Input: part model. Units: mm. Frame: model coordinates. Face numbers are marked on the shaded views. A direction names the side the tool comes from. Coordinates: 2 decimals unless noted, no trailing zeros. Write each loop counter-clockwise with the first axis right and the second up, starting at its lowest first coordinate (ties: lowest second). Pieces come first, ordered by that corner, then holes. Notation, with made-up numbers: (17, 70.25) -> (21, 70.25) arc R11 cw to (21, 91.25) -> close; hole circle Ø8 at (87.5, 30). An arc over 180 degrees is marked (long way). Use one line per item in the form item = value. Start each with the question number.
(1) Ray query, line 1 along Z through (x, y) = (0.05, -24.13) (3 decimals); line 2 along X through (y, z) = (-22.5, 2); line 3 along Y through (x, z) = (2.25, 0.75). Return the intervals inside material, ascending.
(2) Set-up query: the marked faces 1, 2, 3, 4 and 5. Return all of +Z, -Z, +X, -X, +Y, -Y with unobstructed straight access to the full face (end or side cutting, diameter ignored); none if empty.
(3) Cut plane B-B on x = -1.25. Return the cut outline in (y, z) (3 decimals), plus the area to 3 significant figures.
(4) Cut plane C-C on z = -1. Return the cut outline in (x, y), plus the area to 3 significant figures.
(5) Cut plane D-D on y = -9.5. Return the cut outline in (x, z).
(6) First-contact query: pin 1 (1.5 mm diameter, centred on y = -24.13, z = 0, fed in from +X); pin 2 (1.6 mm diameter, centred on y = -21, z = 0, fed in from -X); pin 3 (1 mm diameter, centred on x = 0, z = 3.5, fed in from -Y). Flat tips, straight axial feed; report the tip coordinate or a pass-through.
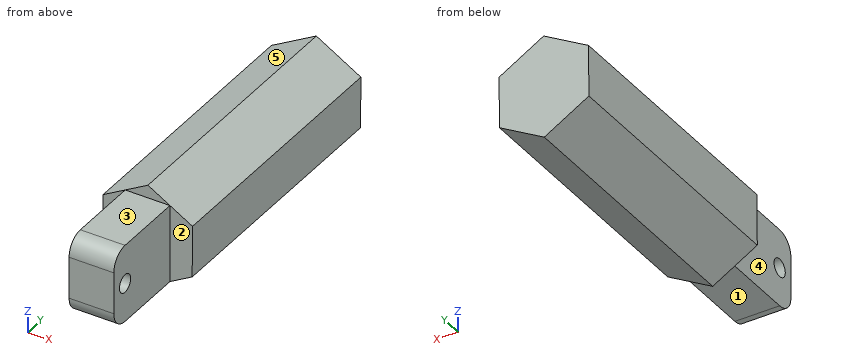
```python
from build123d import *

# Parameters (mm, degrees)
F1_DEPTH = 19.05
F2_W     = 3.175
F2_H     = 5.499398
F3_DEPTH = 6.35
F4_R     = 1.27
F6_D     = 1.27
F6_DEPTH = 25.4


with BuildPart() as f1:
    # F0 (on Front) → F1 (new body)
    with BuildSketch(Plane.XZ):
        Polygon((3.186096, 1.813733), (0.022309, 3.666106), (-3.163787, 1.852373), (-3.186096, -1.813733), (-0.022309, -3.666106), (3.163787, -1.852373), align=None)
    extrude(amount=F1_DEPTH)

    # F2 (on face) → F3 (join)
    with BuildSketch(Plane.XZ.offset(19.05)):
        Rectangle(F2_W, F2_H)
    extrude(amount=F3_DEPTH)

    # F4
    f4_edges = [f1.edges().sort_by_distance(p)[0] for p in [
        (0, -25.4, 2.749699),
        (0, -25.4, -2.749699),
    ]]
    fillet(f4_edges, radius=F4_R)

    # F6
    with Locations(Plane.YZ.offset(1.5875)):
        with Locations((-24.13, 0)):
            Hole(F6_D / 2, depth=F6_DEPTH)


solid = f1.part
```
Values:
q1.line_1 = -2.75 to -0.635, 0.635 to 2.75
q1.line_2 = -1.59 to 1.59
q1.line_3 = -19.05 to 0
q2.face_1 = -Z, +X, -X, -Y
q2.face_2 = +Z, -Z, +X, -Y
q2.face_3 = +Z, +X, -X, -Y
q2.face_4 = +Z, -Z, -X, -Y
q2.face_5 = +Z, -X, +Y, -Y
q3.outline = (-25.4, -1.48) arc R1.27 ccw to (-24.13, -2.75) -> (-19.05, -2.75) -> (-19.05, -2.947) -> (0, -2.947) -> (0, 2.942) -> (-19.05, 2.942) -> (-19.05, 2.75) -> (-24.13, 2.75) arc R1.27 ccw to (-25.4, 1.48) -> close; hole circle Ø1.27 at (-24.13, 0)
q3.area = 145 mm2
q4.outline = (-3.18, -19.05) -> (-1.59, -19.05) -> (-1.59, -25.4) -> (1.59, -25.4) -> (1.59, -19.05) -> (3.17, -19.05) -> (3.17, 0) -> (-3.18, 0) -> close
q4.area = 141 mm2
q5.outline = (-3.19, -1.81) -> (-0.02, -3.67) -> (3.16, -1.85) -> (3.19, 1.81) -> (0.02, 3.67) -> (-3.16, 1.85) -> close
q6.pin_1 = 1.59
q6.pin_2 = -1.59
q6.pin_3 = -19.05
